Answer from the drawing. Dimensions are ordinates in mm from the lowest x, y and z of the part. Give positions to 0.01 mm unless a question says otherwise; leave off trailing zeros. Loops run counter-clockwise (first coordinate to the right, second up) from the corner with the lowest first, then second, coordinate; pieces in that order, holes last. Notation, with made-up numbers: M 45.5,8.25 L 61.5,8.25 A23 cw 61.5,23.25 Z; hole C 18.25,1.5 d5. An arc over 180 degrees is marked long. Return JSON: item names as keys, results as strings. Group by question number.
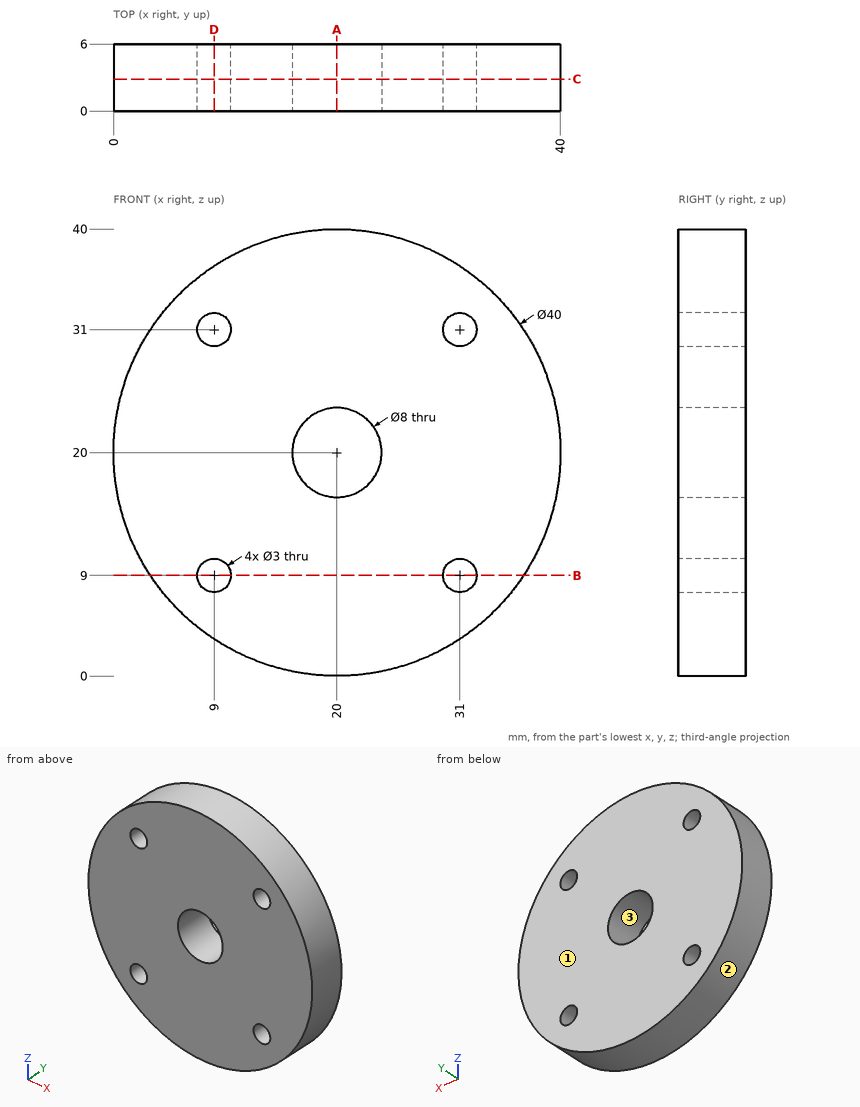
1. Flat-ended cylindrical pins translate along their axes: P1, Ø1, axis at x = 25, y = 1, coming from the +Z side; P2, Ø1.5, axis at y = 2, z = 13, coming from the -X side; P3, Ø1, axis at x = 6.5, y = 1, coming from the -Z side. Find the tip coordinate at first contact, or state that the pin passes through.
2. Find section D-D (x = 9). Write down the section's boundary in (y, z).
3. The mould has two halves that part along Z. Classify the marked faces 1, 2 and 3: +Z half, -Z half, draft (parallel to the pull), parting line (faces both ways), or undercut.
4. Find section A-A (x = 20). Write down the section's boundary in (y, z).
5. Find section C-C (y = 2.85). Write down the section's boundary in (x, z).
6. Straight lines are drawn through the part: line 1 along X through (y, z) = (3.75, 9); line 2 along X through (y, z) = (4.05, 8); line 3 along Z through (x, y) = (30, 0.85). For each, find the intervals that lie inside material, in ascending order.
7. Find section B-B (z = 9). Write down the section's boundary in (x, y).
Result:
{
 "1": {"P1": "stops at z = 39.49", "P2": "stops at x = 1", "P3": "stops at z = 4.8"},
 "2": {"outline": "M 0,3.3 L 6,3.3 L 6,7.5 L 0,7.5 Z; M 0,10.5 L 6,10.5 L 6,29.5 L 0,29.5 Z; M 0,32.5 L 6,32.5 L 6,36.7 L 0,36.7 Z"},
 "3": {"face 1": "draft", "face 2": "parting line", "face 3": "undercut"},
 "4": {"outline": "M 0,0 L 6,0 L 6,16 L 0,16 Z; M 0,24 L 6,24 L 6,40 L 0,40 Z"},
 "5": {"outline": "C 20,20 d40; hole C 9,9 d3; hole C 9,31 d3; hole C 20,20 d8; hole C 31,9 d3; hole C 31,31 d3"},
 "6": {"line 1": "x = 3.3 to 7.5, 10.5 to 29.5, 32.5 to 36.7", "line 2": "x = 4 to 7.88, 10.12 to 29.88, 32.12 to 36", "line 3": "z = 2.68 to 7.88, 10.12 to 29.88, 32.12 to 37.32"},
 "7": {"outline": "M 3.3,0 L 7.5,0 L 7.5,6 L 3.3,6 Z; M 10.5,0 L 29.5,0 L 29.5,6 L 10.5,6 Z; M 32.5,0 L 36.7,0 L 36.7,6 L 32.5,6 Z"}
}
